Build history of the part. All positions in model axes, mm. A direction names the side the tool comes from. Give positions to 0.01 mm unless a question says otherwise; leave off trailing zeros. Write each loop counter-clockwise with the first axis right and the second up, starting at its lowest first coordinate (ties: lowest second). Pieces come first, ordered by that corner, then holes.
from build123d import *

# Parameters (mm, degrees)
BOSS_EXTRUDE2_DEPTH = 71.12
CUT_EXTRUDE1_DEPTH  = 180.537265516
SKETCH6_3_R         = 6.35
CUT_EXTRUDE2_DEPTH  = 180.537265516


with BuildPart() as part:
    # Sketch1 → Boss-Extrude2 (new body)
    with BuildSketch(Plane(origin=(0, 0, 0), x_dir=(0, 0, -1), z_dir=(1, 0, 0))):
        with BuildLine():
            Line((33.224679849, 0), (-33.224679849, 0))
            ThreePointArc((-33.224679849, 0), (-44.45, 4.649679849), (-49.099679849, 15.875))
            Line((-49.099679849, 15.875), (-49.099679849, 132.4102))
            Line((-49.099679849, 132.4102), (-41.149479849, 132.4102))
            Line((-41.149479849, 132.4102), (-41.149479849, 15.9004))
            ThreePointArc((-41.149479849, 15.9004), (-38.82092018, 10.278759668), (-33.199279849, 7.9502))
            Line((-33.199279849, 7.9502), (33.199279849, 7.9502))
            ThreePointArc((33.199279849, 7.9502), (38.82092018, 10.278759668), (41.149479849, 15.9004))
            Line((41.149479849, 15.9004), (41.149479849, 132.4102))
            Line((41.149479849, 132.4102), (49.099679849, 132.4102))
            Line((49.099679849, 132.4102), (49.099679849, 15.875))
            ThreePointArc((49.099679849, 15.875), (44.45, 4.649679849), (33.224679849, 0))
        make_face()
    extrude(amount=BOSS_EXTRUDE2_DEPTH)

    # Sketch6 → Cut-Extrude1 (cut, through all)
    with BuildSketch(Plane.XY.offset(49.099679849)):
        with BuildLine():
            Line((71.12, 132.4102), (35.56, 132.4102))
            ThreePointArc((35.56, 132.4102), (60.704717139, 121.994917139), (71.12, 96.8502))
            Line((71.12, 96.8502), (71.12, 132.4102))
        make_face()
        with BuildLine():
            Line((0, 132.4102), (0, 96.8502))
            ThreePointArc((0, 96.8502), (10.415282861, 121.994917139), (35.56, 132.4102))
            Line((35.56, 132.4102), (0, 132.4102))
        make_face()
    extrude(amount=-CUT_EXTRUDE1_DEPTH, mode=Mode.SUBTRACT)

    # Sketch6_3 → Cut-Extrude2 (cut, through all)
    with BuildSketch(Plane.XY.offset(49.099679849)):
        with Locations((35.56, 96.8502)):
            Circle(SKETCH6_3_R)
    extrude(amount=-CUT_EXTRUDE2_DEPTH, mode=Mode.SUBTRACT)


solid = part.part
1. Mould opens along Y. For faces 1 (the face through (34.18, 90.65, -45.07)), 2 (the face through (35, 0, 0)), 3 (the face through (0, 6, 0)) say: pulls with the +Y half, pulls with the -Y half, needs draft (parallel to the pull), parting line crosses it, or undercut.
2. Saw through at D-D on x = 66. Give the cut face in (y, z) (3 decimals).
3. Saw through at B-B on y = 14. Give the cut face in (x, z), plus the area to 3 significant figures.
4. 3-axis set-ups, long thin cutter, end or side, ignore diameter. For faces 4 (the face through (35, 73, 49.1)), 5 (the face through (35, 75, 41.149)): which of +Z, -Z, +X, -X, +Y, -Y reach the whole face in a straight line?
5. Drop flat-ended pins along their axis: pin 1 (1.5 mm diameter, centred on x = 59.5, z = -1.5, fed in from +Y); pin 2 (1 mm diameter, centred on x = 10.5, z = -35.5, fed in from -Y); pin 3 (2 mm diameter, centred on x = 48.5, z = 33.5, fed in from +Y). Give the stop position or say it passes through.
6. Drill centre lines: line 1 along Z through (x, y) = (43, 61); line 2 along Y through (x, z) = (15, 0.5); line 3 along Y through (x, z) = (35, 45). Where is each one in solid material? Low to high.
7. Saw through at C-C on z = -31. Give the cut face in (x, y).
8. Saw through at A-A on x = 38. Give the cut face in (y, z) (3 decimals), plus the area to 3 significant figures.
Outcome:
1. face 1: undercut
1. face 2: pulls with the -Y half
1. face 3: needs draft
2. outline: (0, -33.225) arc R15.875 ccw to (15.875, -49.1) - (115.233, -49.1) - (115.233, -41.149) - (15.9, -41.149) arc R7.95 cw to (7.95, -33.199) - (7.95, 33.199) arc R7.95 cw to (15.9, 41.149) - (115.233, 41.149) - (115.233, 49.1) - (15.875, 49.1) arc R15.875 ccw to (0, 33.225) - close
3. outline: (0, -48.99) - (71.12, -48.99) - (71.12, -40.92) - (0, -40.92) - close; (0, 40.92) - (71.12, 40.92) - (71.12, 48.99) - (0, 48.99) - close
3. area: 1,150 mm2
4. face 4: +Z, +X, -X, +Y, -Y
4. face 5: +X, -X, +Y
5. pin 1: stops at y = 7.95
5. pin 2: stops at y = 0.1
5. pin 3: stops at y = 8.06
6. line 1: z = -49.1 to -41.15, 41.15 to 49.1
6. line 2: y = 0 to 7.95
6. line 3: y = 5.23 to 90.52, 103.18 to 132.41
7. outline: (0, 0) - (71.12, 0) - (71.12, 7.95) - (0, 7.95) - close
8. outline: (0, -33.225) arc R15.875 ccw to (15.875, -49.1) - (90.988, -49.1) - (90.988, -41.149) - (15.9, -41.149) arc R7.95 cw to (7.95, -33.199) - (7.95, 33.199) arc R7.95 cw to (15.9, 41.149) - (90.988, 41.149) - (90.988, 49.1) - (15.875, 49.1) arc R15.875 ccw to (0, 33.225) - close; (102.713, -49.1) - (132.326, -49.1) - (132.326, -41.149) - (102.713, -41.149) - close; (102.713, 41.149) - (132.326, 41.149) - (132.326, 49.1) - (102.713, 49.1) - close
8. area: 2,490 mm2
